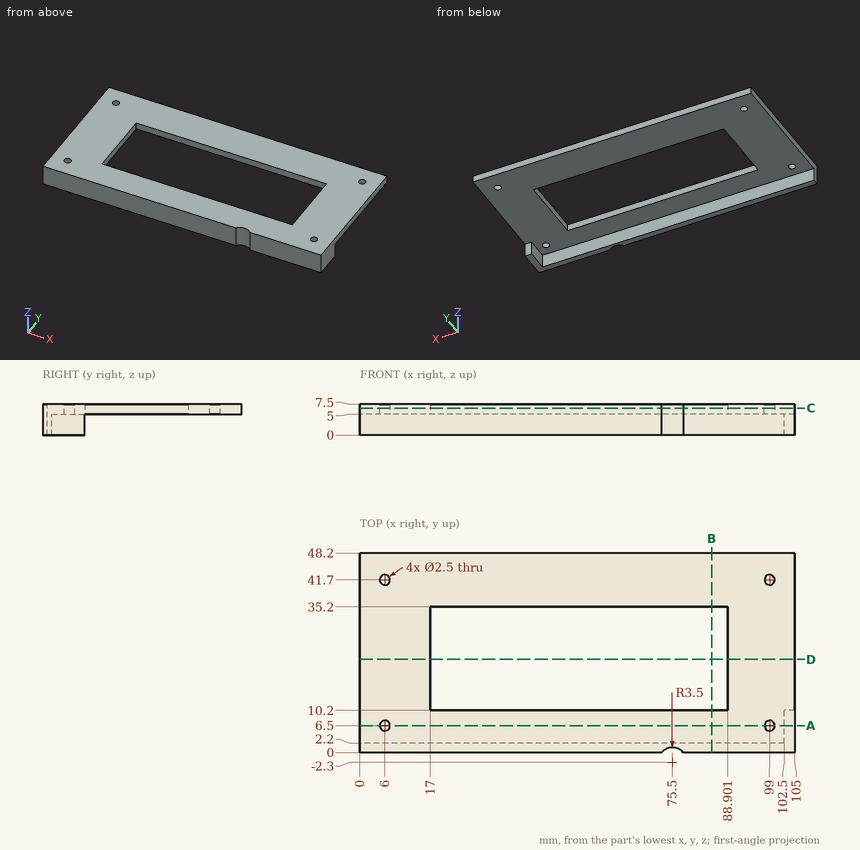
Drawing for the job (mm, zero at the part's lowest x, y, z). Round coordinates to 2 decimals unless told otherwise and drop trailing zeros. Write each loop counter-clockwise with the first axis right and the second up, starting at its lowest first coordinate (ties: lowest second). Pieces come first, ordered by that corner, then holes. Notation, with made-up numbers: M -26.5,89 L 9.5,89 A14 ccw 9.5,103 Z; hole C 27.25,56 d1. An arc over 180 degrees is marked long. Answer as a JSON object with one key per item and string values. Group by question number.
(1) Cut at A-A (y = 6.5). Give the cut face in (x, z).
(2) Drill centre lines: L1, parallel to Y at x = 99, z = 5.85; L2, parallel to Y at x = 57.5, z = 5.25; L3, parallel to X at y = 41.7, z = 6.1. Where is each one in solid material? Low to high.
(3) Cut at D-D (y = 22.5). Give the cut face in (x, z).
(4) Cut at B-B (x = 85). Give the cut face in (y, z), and give its area (3 significant figures).
(5) Cut at C-C (z = 6.5). Give the cut face in (x, y), and give its area (3 significant figures).
(6) Flat gauge pins, fed straight in: pin 1 (6 mm diameter, centred on x = 48, y = 37.5, fed in from -Z); pin 2 (1.5 mm diameter, centred on x = 58.5, z = 2.5, fed in from +Y); pin 3 (2.5 mm diameter, centred on y = 4.5, z = 2.5, fed in from -X); pin 4 (2 mm diameter, centred on x = 6, y = 41.7, fed in from +Z). Where does each tip first touch, or does it go through?
Responses:
{
 "1": {"outline": "M 0,5 L 4.75,5 L 4.75,7.5 L 0,7.5 Z; M 7.25,5 L 97.75,5 L 97.75,7.5 L 7.25,7.5 Z; M 100.25,5 L 102.5,5 L 102.5,0 L 105,0 L 105,7.5 L 100.25,7.5 Z"},
 "2": {"L1": "y = 0 to 5.25, 7.75 to 40.45, 42.95 to 48.2", "L2": "y = 0 to 10.2, 35.2 to 48.2", "L3": "x = 0 to 4.75, 7.25 to 97.75, 100.25 to 105"},
 "3": {"outline": "M 0,5 L 17,5 L 17,7.5 L 0,7.5 Z; M 88.9,5 L 105,5 L 105,7.5 L 88.9,7.5 Z"},
 "4": {"outline": "M 0,0 L 2.2,0 L 2.2,5 L 10.2,5 L 10.2,7.5 L 0,7.5 Z; M 35.2,5 L 48.2,5 L 48.2,7.5 L 35.2,7.5 Z", "area": "69.0 mm2"},
 "5": {"outline": "M 0,0 L 72.86,0 A3.5 cw 78.14,0 L 105,0 L 105,48.2 L 0,48.2 Z; hole C 6,6.5 d2.5; hole C 6,41.7 d2.5; hole M 17,10.2 L 88.9,10.2 L 88.9,35.2 L 17,35.2 Z; hole C 99,6.5 d2.5; hole C 99,41.7 d2.5", "area": "3,240 mm2"},
 "6": {"pin 1": "stops at z = 5", "pin 2": "stops at y = 2.2", "pin 3": "stops at x = 102.5", "pin 4": "passes through"}
}
